Can you work these out from the model? Positions are in its coordinate system, mm. A direction names the side the tool comes from. Give positions to 0.01 mm unless a question says otherwise; leave off trailing zeros. Loops run counter-clockwise (first coordinate to the right, second up) from the corner with the lowest first, then second, coordinate; pieces in that order, holes last. Notation, with made-up numbers: (7, -11.75) -> (59, -11.75) arc R23 cw to (59, 24.25) -> close; hole circle Ø3 at (-3.5, 11.5). An arc over 180 degrees is marked (long way). One line per question, with ' | ' between items.
from build123d import *

# Parameters (mm, degrees)
SKETCH3_W                   = 152.4
SKETCH3_H                   = 22.225
BOSS_EXTRUDE1_DEPTH         = 76.2
M3_TAPPED_HOLE1_D           = 2.5
SKETCH10_R                  = 38.1
CUT_EXTRUDE3_DEPTH          = 12.7
M3_TAPPED_HOLE2_D           = 2.5
M3_TAPPED_HOLE2_CSINK_D     = 3.05
M3_TAPPED_HOLE2_CSINK_ANGLE = 90


with BuildPart() as part:
    # Sketch3 → Boss-Extrude1 (new, symmetric)
    with BuildSketch(Plane.XY):
        Rectangle(SKETCH3_W, SKETCH3_H)
    extrude(amount=BOSS_EXTRUDE1_DEPTH, both=True)

    # M3 Tapped Hole1 (through all)
    with Locations(Plane(origin=(0, -11.1125, 0), x_dir=(-1, 0, 0), z_dir=(0, -1, 0))):
        with Locations((-50.8, -23.8125), (50.8, -23.8125)):
            Hole(M3_TAPPED_HOLE1_D / 2)

    # Sketch10 → Cut-Extrude3 (cut)
    with BuildSketch(Plane(origin=(0, 11.1125, 0), x_dir=(1, 0, 0), z_dir=(0, 1, 0))):
        with Locations(Location((0, 30.95625, 0), (0, 0, 270))):
            Circle(SKETCH10_R)
    extrude(amount=-CUT_EXTRUDE3_DEPTH, mode=Mode.SUBTRACT)

    # M3 Tapped Hole2 (through all)
    with Locations(Plane(origin=(0, -11.1125, 0), x_dir=(-1, 0, 0), z_dir=(0, -1, 0))):
        with Locations((0, 30.95625)):
            CounterSinkHole(M3_TAPPED_HOLE2_D / 2, M3_TAPPED_HOLE2_CSINK_D / 2, counter_sink_angle=M3_TAPPED_HOLE2_CSINK_ANGLE)


solid = part.part
Q1. If we section it at C-C (x = -23): Write out the boundary of the cut face in (y, z), plus the area to 3 significant figures.
Entries:
outline: (-11.11, -76.2) -> (11.11, -76.2) -> (11.11, -61.33) -> (-1.59, -61.33) -> (-1.59, -0.58) -> (11.11, -0.58) -> (11.11, 76.2) -> (-11.11, 76.2) -> close | area: 2,620 mm²
Q2. If I drill on probe 1 along Z at (x, y) = (-50.8, 0); probe 2 along Z at (x, y) = (0, -7.5); probe 3 along Y at (x, z) = (30, -20.5), over which ranges is the centre line in solid material (lowest first)? Write a range as from..to.
Entries:
probe 1: -76.2..22.56, 25.06..76.2 | probe 2: -76.2..-32.21, -29.71..76.2 | probe 3: -11.11..-1.59
Q3. If we section it at A-A (y = 7): Write out the boundary of the cut face in (x, z).
Entries:
outline: (-76.2, -76.2) -> (76.2, -76.2) -> (76.2, 76.2) -> (-76.2, 76.2) -> close; hole circle Ø2.5 at (-50.8, 23.81); hole circle Ø76.2 at (0, -30.96); hole circle Ø2.5 at (50.8, 23.81)
Q4. If we mould it in two halves opening along X, with no side actions, what happens to faces 1 (the face through (-1, 0, -76.2)), 2 (the face through (-76.2, 0, 1)), 3 (the face through (11.4, 4.9, 5.4)), 4 (the face through (76.2, 0, 1))? For each: pulls with the +X half, pulls with the -X half, needs draft (parallel to the pull), parting line crosses it, or undercut.
Entries:
face 1: needs draft | face 2: pulls with the -X half | face 3: undercut | face 4: pulls with the +X half
Q5. On a 3-axis mill with a long thin cutter (end or side, diameter ignored), from which of +Z, -Z, +X, -X, +Y, -Y can I reach the whole of each face in a straight line? I mean faces 5 (the face through (-1, -11.112, 1)), 6 (the face through (1, -1.587, -23)). Say none if no direction works.
Entries:
face 5: +Z, -Z, +X, -X, -Y | face 6: +Y
Q6. For pin 1 Ø23 at (x, z) = (-6.5, -35) entering from +Y; pin 2 Ø3 at (x, z) = (50.8, 23.81) entering from +Y, each with a flat end and sliding along its axis, tell me the tip position at first contact or that it passes through.
Entries:
pin 1: y = -1.59 | pin 2: y = 11.11
Q7. If we section it at B-B (z = 0): Write out the boundary of the cut face in (x, y), plus the area to 3 significant figures.
Entries:
outline: (-76.2, -11.11) -> (76.2, -11.11) -> (76.2, 11.11) -> (22.21, 11.11) -> (22.21, -1.59) -> (-22.21, -1.59) -> (-22.21, 11.11) -> (-76.2, 11.11) -> close | area: 2,820 mm²
